```python
from build123d import *

# Parameters (mm, degrees)
REVOLVE2_ANGLE          = 180
CUT_EXTRUDE1_DEPTH      = 6.477
CUT_EXTRUDE1_DEPTH_BACK = 6.477


# Read off the part's stored shape, not the designer's step: Revolve2
with BuildPart() as part:
    # Revolve2 outline → Revolve2 (revolve)
    with BuildSketch(Plane.XZ):
        Polygon((3.81, 0), (0, 0), (0, -3.81), (38.1, -41.91), (41.91, -41.91), (41.91, -38.1), align=None)
    revolve(axis=Axis((0, 0, 0), (0, 0, 1)), revolution_arc=REVOLVE2_ANGLE)

    # Sketch6 → Cut-Extrude1 (cut, two sides: drawn at the far end of the back side and taken through both)
    with BuildSketch(Plane(origin=(0, 0, 0), x_dir=(0, 0, -1), z_dir=(1, 0, 0)).offset(-CUT_EXTRUDE1_DEPTH_BACK)):
        Polygon((19.412948776, 19.412948776), (19.412948776, 29.318948776), (19.412948776, 36.223650293), (29.344348776, 36.223650293), (29.344348776, 29.344348776), align=None)
    extrude(amount=CUT_EXTRUDE1_DEPTH + CUT_EXTRUDE1_DEPTH_BACK, mode=Mode.SUBTRACT)


solid = part.part
```
CAD build for the part. Positions are in the model's coordinates, mm. A direction names the side the tool comes from. Round coordinates to 2 decimals unless told otherwise and drop trailing zeros. Write each loop counter-clockwise with the first axis right and the second up, starting at its lowest first coordinate (ties: lowest second). Pieces come first, ordered by that corner, then holes. Notation, with made-up numbers: (-2, 54.25) -> (17, 54.25) arc R23 ccw to (17, 70.25) -> close; hole circle Ø5 at (73, 89.25). An arc over 180 degrees is marked (long way). Answer in a Markdown table with one row per item. Add a question column.
Item 1: Drop flat-ended pins along their axis: pin 1 Ø6 at (x, y) = (-20, 13) entering from -Z; pin 2 Ø8 at (y, z) = (27, -26) entering from +X; pin 3 Ø1.1 at (x, y) = (-1, 31) entering from +Z. Give the stop position or say it passes through.
Item 2: Saw through at B-B, the plane z = -15. Write the cut outline in (x, y), then the cut area to 3 significant figures.
Item 3: Mould opens along X. For faces 4 (the face through (0.9, 41.9, -40)), 5 (the face through (-6.477, 26, -24)), 6 (the face through (0, 2, 0)) say: pulls with the +X half, pulls with the -X half, needs draft (parallel to the pull), parting line crosses it, or undercut.
Item 4: Saw through at A-A, the plane x = 0. Write the cut outline in (y, z), then the cut area to 3 significant figures.
Item 5: Drill centre lines: line 1 (X direction, y = 31, z = -40); line 2 (X direction, y = 4, z = -8.5); line 3 (Z direction, x = 32, y = 19). Where is each one in solid material? Low to high. Write a range as from..to.
Item 6: Saw through at C-C, the plane z = -22. Write the cut outline in (x, y).
Item 7: Which spindle directions (+Z, -Z, +X, -X, +Y, -Y) get a long thin tool onto all of the face, cutting with end or side? Do faces 1 (the face through (0, 24, -24)), 2 (the face through (0, 31, -29.344)), 3 (the face through (0.332, 15.08, -18.893)). Say none if no direction does.
Findings below:
| question | item | result |
|---|---|---|
| 1 | pin 1 | stops at z = -30.66 |
| 1 | pin 2 | stops at x = 22.01 |
| 1 | pin 3 | stops at z = -29.34 |
| 2 | outline | (-18.81, 0) -> (-11.19, 0) arc R11.19 cw to (11.19, 0) -> (18.81, 0) arc R18.81 ccw to start |
| 2 | area | 359 mm^2 |
| 3 | face 4 | parting line crosses it |
| 3 | face 5 | undercut |
| 3 | face 6 | needs draft |
| 4 | outline | (0, -3.81) -> (38.1, -41.91) -> (41.91, -41.91) -> (41.91, -38.1) -> (33.15, -29.34) -> (29.34, -29.34) -> (19.41, -19.41) -> (23.22, -19.41) -> (3.81, 0) -> (0, 0) -> close |
| 4 | area | 267 mm^2 |
| 5 | line 1 | x = -28.2..-18.67, 18.67..28.2 |
| 5 | line 2 | x = -11.64..-2.45, 2.45..11.64 |
| 5 | line 3 | z = -41.03..-33.41 |
| 6 | outline | (-25.81, 0) -> (-18.19, 0) arc R18.19 cw to (18.19, 0) -> (25.81, 0) arc R25.81 ccw to (6.48, 24.98) -> (6.48, 22) -> (-6.48, 22) -> (-6.48, 24.98) arc R25.81 ccw to start |
| 7 | face 1 | +Y |
| 7 | face 2 | +Z, +Y |
| 7 | face 3 | -Z, -Y |
